Design review of the part shown in the three views and the two pictorial views. Dimensions are in mm from the part's minimum x, y and z. A direction names the side the tool comes from. Coordinates: 2 decimals unless noted, no trailing zeros. Loops run counter-clockwise (first coordinate to the right, second up) from the corner with the lowest first, then second, coordinate; pieces in that order, holes last. Notation, with made-up numbers: (22.5, 19) -> (29.5, 19) arc R26 cw to (29.5, 48) -> close; hole circle Ø4 at (33.25, -19.75). An arc over 180 degrees is marked (long way). One line per item, written item: value. Start each with the question number.
1. Add section A-A on z = 9.3. Write out the cut boundary in (x, y), plus the area to 3 significant figures.
2. Machinability: for the marked faces 4 and 5, which of the approach directions +Z, -Z, +X, -X, +Y, -Y give a long, thin tool a straight path to every point of the face, cutting with its end or side? Answer none if there is none.
3. Draft analysis for pull direction X (two halves, no side actions). For the marked faces 1, 2 and 3, state which applies: pulls with the +X half, pulls with the -X half, needs draft (parallel to the pull), parting line crosses it, or undercut.
4. Insertion check: pin 1 (6 mm diameter, centred on y = 5.5, z = 16.5, fed in from -X); pin 2 (8 mm diameter, centred on y = 16, z = 14.5, fed in from +X); pin 3 (4 mm diameter, centred on x = 6, y = 13, fed in from +Z). Each pin has a flat end and moves straight along its axis. Give the tip position at first contact, or say it passes through.
5. For probe 1 along X at (y, z) = (3.5, 9.25); probe 2 along Y at (x, z) = (7.75, 11.5), list the stretches that pass through material, from the lowest coordinate up.
6. Add section B-B on y = 7.75. Write out the cut boundary in (x, z), plus the area to 3 significant figures.
7. Add section D-D on y = 11.5. Write out the cut boundary in (x, z), plus the area to 3 significant figures.
8. Add section C-C on x = 9.3. Write out the cut boundary in (y, z), plus the area to 3 significant figures.
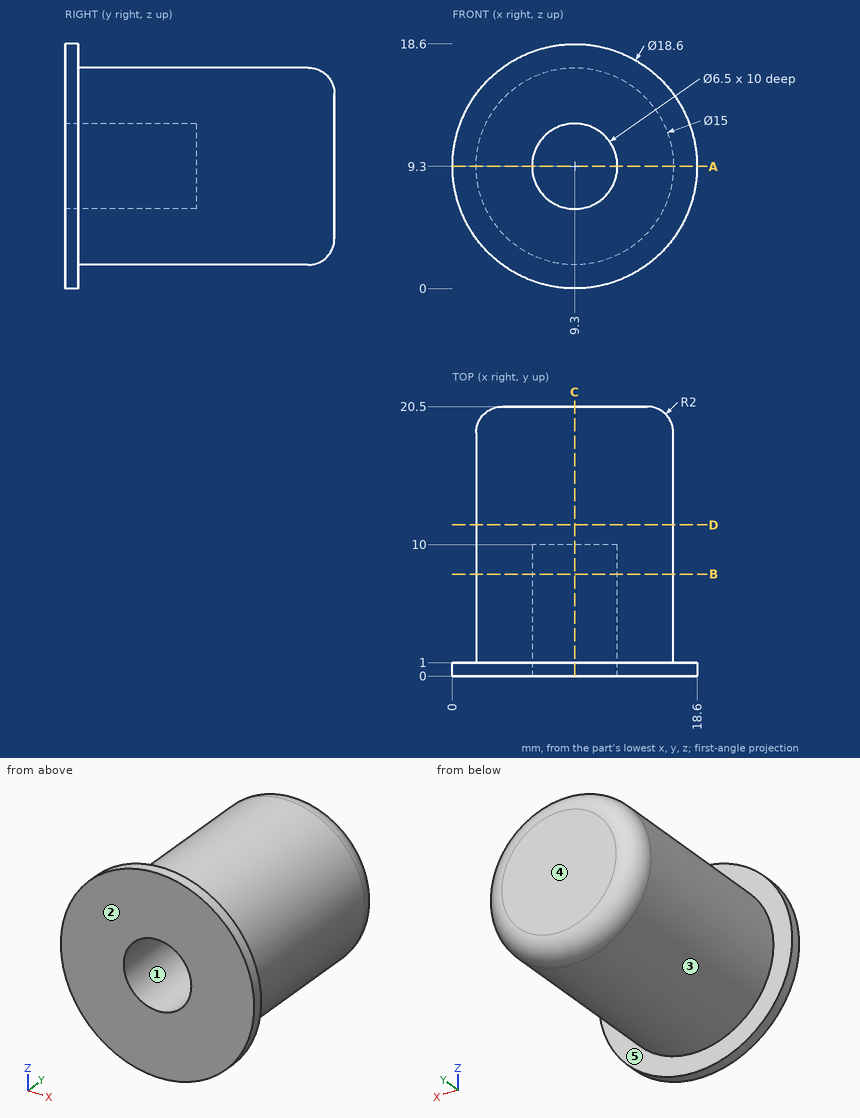
Worked answers:
1. outline: (0, 0) -> (6.05, 0) -> (6.05, 10) -> (12.55, 10) -> (12.55, 0) -> (18.6, 0) -> (18.6, 1) -> (16.8, 1) -> (16.8, 18.5) arc R2 ccw to (14.8, 20.5) -> (3.8, 20.5) arc R2 ccw to (1.8, 18.5) -> (1.8, 1) -> (0, 1) -> close
1. area: 244 mm²
2. face 4: +Z, -Z, +X, -X, +Y
2. face 5: +Y
3. face 1: undercut
3. face 2: needs draft
3. face 3: parting line crosses it
4. pin 1: stops at x = 3.09
4. pin 2: stops at x = 16.7
4. pin 3: stops at z = 16.69
5. probe 1: x = 1.8 to 6.05, 12.55 to 16.8
5. probe 2: y = 10 to 20.5
6. outline: circle Ø15 at (9.3, 9.3); hole circle Ø6.5 at (9.3, 9.3)
6. area: 144 mm²
7. outline: circle Ø15 at (9.3, 9.3)
7. area: 177 mm²
8. outline: (0, 0) -> (1, 0) -> (1, 1.8) -> (18.5, 1.8) arc R2 ccw to (20.5, 3.8) -> (20.5, 14.8) arc R2 ccw to (18.5, 16.8) -> (1, 16.8) -> (1, 18.6) -> (0, 18.6) -> (0, 12.55) -> (10, 12.55) -> (10, 6.05) -> (0, 6.05) -> close
8. area: 244 mm²
